Check sheet for the modelled part. Datum: model origin and axes. Units: mm. Give positions to 0.01 mm unless a question says otherwise; leave off trailing zeros. Order: outer loops, then holes, each group sorted by start corner. A loop starts at its lowest first (then second) coordinate and runs counter-clockwise, first axis right, second up.
```python
from build123d import *

# Parameters (mm, degrees)
SKETCH1_W           = 90
SKETCH1_H           = 160
BOSS_EXTRUDE1_DEPTH = 2
SKETCH2_W           = 20
SKETCH2_H           = 10
BOSS_EXTRUDE2_DEPTH = 1
LPATTERN1_COUNT     = 3
LPATTERN1_PITCH     = 30
FILLET1_R           = 2


with BuildPart() as part:
    # Sketch1 → Boss-Extrude1 (new body)
    with BuildSketch(Plane(origin=(0, 0, 0), x_dir=(1, 0, 0), z_dir=(0, 1, 0))):
        Rectangle(SKETCH1_W, SKETCH1_H)
    extrude(amount=BOSS_EXTRUDE1_DEPTH)

    # Sketch2 → Boss-Extrude2 (add)
    with BuildSketch(Plane(origin=(0, 2, 0), x_dir=(1, 0, 0), z_dir=(0, 1, 0))):
        with Locations((-30, 70)):
            Rectangle(SKETCH2_W, SKETCH2_H)
        with Locations((-30, 55)):
            Rectangle(SKETCH2_W, SKETCH2_H)
        with Locations((-30, 40)):
            Rectangle(SKETCH2_W, SKETCH2_H)
        with Locations((-30, 25)):
            Rectangle(SKETCH2_W, SKETCH2_H)
        with Locations((-30, 10)):
            Rectangle(SKETCH2_W, SKETCH2_H)
        with Locations((-30, -5)):
            Rectangle(SKETCH2_W, SKETCH2_H)
        with Locations((-30, -20)):
            Rectangle(SKETCH2_W, SKETCH2_H)
        with Locations((-30, -35)):
            Rectangle(SKETCH2_W, SKETCH2_H)
        with Locations((-30, -50)):
            Rectangle(SKETCH2_W, SKETCH2_H)
        with Locations((-30, -65)):
            Rectangle(SKETCH2_W, SKETCH2_H)
    boss_extrude2 = extrude(amount=BOSS_EXTRUDE2_DEPTH)

    # LPattern1: Boss-Extrude2 ×3
    with Locations(*[(i * LPATTERN1_PITCH, 0, 0) for i in range(1, LPATTERN1_COUNT)]):
        add(boss_extrude2)

    # Fillet1
    fillet1_edges = [part.edges().sort_by_distance(p)[0] for p in [
        (-45, 1, -80),
        (45, 1, -80),
        (45, 1, 80),
        (-45, 1, 80),
    ]]
    fillet(fillet1_edges, radius=FILLET1_R)


solid = part.part
```
(1) Cross-section at A-A on z = 31.5. Enter the section's corners in (x, y), then the cut area to 3 significant figures.
Response values:
outline: (-45, 0) - (45, 0) - (45, 2) - (40, 2) - (40, 3) - (20, 3) - (20, 2) - (10, 2) - (10, 3) - (-10, 3) - (-10, 2) - (-20, 2) - (-20, 3) - (-40, 3) - (-40, 2) - (-45, 2) - close
area: 240 mm2
(2) Release check for a two-part mould opening along X. For faces 1 (the face through (-11, 2, -1)), 2 (the face through (30, 3, -40)) record: released by +X, released by -X, zero draft, split by the parting line, or undercut.
Response values:
face 1: undercut
face 2: zero draft
(3) Material ranges on L1, parallel to X at y = 2.95, z = 38.5; L2, parallel to Y at x = 10.5, z = 72.5, recorded low to high.
Response values:
L1: x = -40 to -20, -10 to 10, 20 to 40
L2: y = 0 to 2
(4) Gauge pin test, flat ends, axial feed: pin 1 Ø1.1 at (y, z) = (2.5, 20.5) entering from -X; pin 2 Ø0.8 at (y, z) = (2.5, -70) entering from +X; pin 3 Ø4 at (x, z) = (-16.5, 37.5) entering from +Y; pin 4 Ø0.8 at (y, z) = (2.5, 36.5) entering from -X. Record the tip position at first contact, or that the pin passes through.
Response values:
pin 1: stops at x = -45
pin 2: stops at x = 40
pin 3: stops at y = 2
pin 4: stops at x = -40
